Check sheet for the modelled part. Datum: model origin and axes. Units: mm. Face numbers are marked on the shaded views. A direction names the side the tool comes from. Give positions to 0.01 mm unless a question says otherwise; leave off trailing zeros. Write each loop counter-clockwise with the first axis right and the second up, starting at its lowest first coordinate (ties: lowest second). Pieces come first, ordered by that corner, then holes. Notation, with made-up numbers: (62.5, 33) -> (95.5, 33) arc R20 cw to (95.5, 39) -> close; hole circle Ø10 at (17.5, 32.5). An arc over 180 degrees is marked (long way). Use a Markdown table: item, result. Add a question column.
1. Cross-section at D-D (y = -8). Enter the section's corners in (x, z).
2. Cross-section at A-A (y = -1.5). Enter the section's corners in (x, z).
3. Cross-section at B-B (x = 11.5). Enter the section's corners in (y, z).
4. Set-up check for the marked faces 4 and 5: record each of +Z, -Z, +X, -X, +Y, -Y from which the full face is reachable in a straight line by a thin tool's end or side.
5. Cross-section at C-C (z = 5). Enter the section's corners in (x, y), then the cut area to 3 significant figures.
6. Gauge pin test, flat ends, axial feed: P1, Ø2.5, axis at x = 16.5, y = -4.5, coming from the +Z side; P2, Ø6, axis at x = 11.5, z = 6, coming from the +Y side; P3, Ø3.5, axis at y = -4.5, z = 10.5, coming from the +X side. Record the tip position at first contact, or that the pin passes through.
7. Release check for a two-part mould opening along X. For the marked faces 1, 2 and 3 record: released by +X, released by -X, zero draft, split by the parting line, or undercut.
8. Scan lines: probe 1 along Y at (x, z) = (3.2, 10.5); probe 2 along X at (y, z) = (-4.5, 0.95); probe 3 along Z at (x, y) = (8, -0.75). Record each from-to range of solid material in increasing order. Write a range as [from, to].
from build123d import *

# Parameters (mm, degrees)
F1_DEPTH = 9
F2_R     = 1.6
F3_DEPTH = 25
F4_R     = 1.6
F5_DEPTH = 25
F6_R     = 4.49999
F7_ANGLE = 90


# Not quite as in the source:
# - a fillet or chamfer is up to 0.001 mm smaller than in the source, because OpenCascade refuses the exact size


with BuildPart() as f1:
    # F0 (on Front) → F1 (new body)
    with BuildSketch(Plane.XZ):
        Polygon((-15, 4), (-15, 0), (0, 0), (0, 21), (-4, 21), (-4, 4), align=None)
    extrude(amount=F1_DEPTH)

    # F2 (on face) → F3 (cut)
    with BuildSketch(Plane.XY.offset(4)):
        with Locations((-10.5, -4.5)):
            Circle(F2_R)
    extrude(amount=-F3_DEPTH, mode=Mode.SUBTRACT)

    # F4 (on face) → F5 (cut)
    with BuildSketch(Plane(origin=(-4, 0, 0), x_dir=(0, -1, 0), z_dir=(-1, 0, 0))):
        with Locations((4.5, 16.5)):
            Circle(F4_R)
    extrude(amount=-F5_DEPTH, mode=Mode.SUBTRACT)

    # F6 (radius 4.5 in the source; OpenCascade refuses exactly that, so slightly less here)
    f6_edges = [f1.edges().sort_by_distance(p)[0] for p in [
        (-2, -9, 21),
        (-2, 0, 21),
        (-15, 0, 2),
        (-15, -9, 2),
    ]]
    fillet(f6_edges, radius=F6_R)


with BuildPart() as f1_1:
    # F7: moved
    add(f1.part.rotate(Axis((0, -4.5, 0), (0, 1, 0)), F7_ANGLE))


solid = f1_1.part
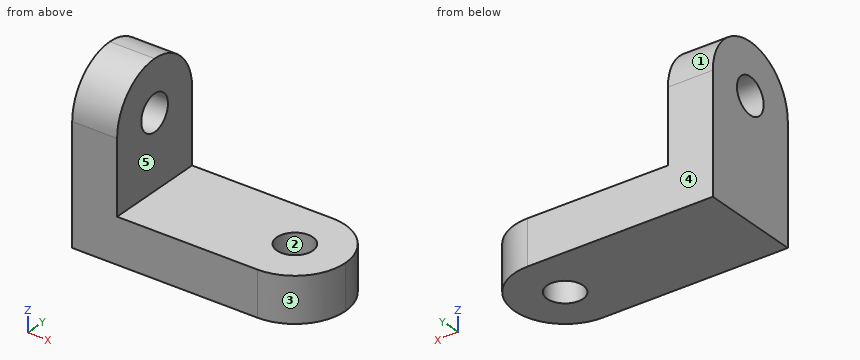
Worked answers:
| question | item | result |
|---|---|---|
| 1 | outline | (0, 0) -> (19.33, 0) -> (19.33, 4) -> (4, 4) -> (4, 13.33) -> (0, 13.33) -> close |
| 2 | outline | (0, 0) -> (19.85, 0) -> (19.85, 4) -> (4, 4) -> (4, 13.85) -> (0, 13.85) -> close |
| 3 | outline | (-9, 0) -> (0, 0) -> (0, 4) -> (-9, 4) -> close |
| 4 | face 4 | +Z, -Z, +X, -X, +Y |
| 4 | face 5 | +Z, +X, +Y, -Y |
| 5 | outline | (0, -9) -> (4, -9) -> (4, 0) -> (0, 0) -> close |
| 5 | area | 36.0 mm² |
| 6 | P1 | passes through |
| 6 | P2 | stops at y = 0 |
| 6 | P3 | stops at x = 4 |
| 7 | face 1 | zero draft |
| 7 | face 2 | undercut |
| 7 | face 3 | released by +X |
| 8 | probe 1 | y = [-9, -6.1], [-2.9, 0] |
| 8 | probe 2 | x = [0, 14.9], [18.1, 21] |
| 8 | probe 3 | z = [0, 4] |
